Design review of the part built by this model. Coordinates are the model's own, in mm. A direction names the side the tool comes from. Round coordinates to 2 decimals unless told otherwise and drop trailing zeros. Write each loop counter-clockwise with the first axis right and the second up, starting at its lowest first coordinate (ties: lowest second). Pieces come first, ordered by that corner, then holes. Notation, with made-up numbers: (74.25, 4.5) -> (120.25, 4.5) arc R20 ccw to (120.25, 22.5) -> close; hole circle Ø1 at (-18, -6.5). An arc over 180 degrees is marked (long way). Write item = value, one per line. Start each with the question number.
Item 1: For pin 1 Ø1 at (x, z) = (2.5, -11.5) entering from +Y; pin 2 Ø3 at (y, z) = (7, 3.5) entering from +X (3 decimals); pin 3 Ø5 at (y, z) = (-9, 4.5) entering from -X; pin 4 Ø4 at (x, z) = (9.5, 15) entering from +Y, all flat-tipped, find the tip position at first contact; note any pin that passes through.
Item 2: Add section D-D, the plane x = -9. State how many separate pieces and enclosed holes the cut face has, then the cut area to 3 significant figures.
Item 3: Mouldability with a two-part tool opening along Y and no side actions: class faces 1 (the flat face through (0, 0, 21)), 2 (the flat face through (1, -8, 0)), 3 (the cylindrical face through (11.923, 3.755, 0.098)) as released by +Y, released by -Y, zero draft, split by the parting line, or undercut.
Item 4: Machinability: for faces 4 (the flat face through (-2, 4, -14.7)), 5 (the flat face through (-8, 1, 0)), 6 (the cylindrical face through (-4.296, 0.189, 17.894)), which of the approach directions +Z, -Z, +X, -X, +Y, -Y give a long, thin tool a straight path to every point of the face, cutting with its end or side? Answer none if there is none.
Item 5: Add section A-A, the plane z = 5. State the section outline as (x, y) points.
Item 6: To check wall thickness, follow L1, parallel to X at y = -4.5, z = 5; L2, parallel to X at y = -7, z = 2; L3, parallel to Y at x = 0.5, z = -3. State the ranges of each line that lie inside material, in increasing order.
Item 7: Add section B-B, the plane x = 0. State the section outline as (y, z) points, then the cut area to 3 significant figures.
from build123d import *

# Parameters (mm, degrees)
F0_R     = 4.3
F0_R_2   = 2.3
F1_DEPTH = 21
F0_R_3   = 12.5
F2_DEPTH = 14.7


with BuildPart() as f1:
    # F0 (on Top) → F1 (new body, symmetric)
    with BuildSketch(Plane.XY):
        Circle(F0_R)
        Circle(F0_R_2, mode=Mode.SUBTRACT)
        Circle(F0_R_2)
    extrude(amount=F1_DEPTH, both=True)

    # F0 (on Top) → F2 (join, symmetric)
    with BuildSketch(Plane.XY):
        Circle(F0_R_3)
        with BuildLine():
            ThreePointArc((1, 10.4522724802), (7.4246212025, 7.4246212025), (10.4522724802, 1))
            ThreePointArc((10.4522724802, 1), (10.4880613328, 0.5005691551), (10.5, 0))
            ThreePointArc((10.5, 0), (10.4880613328, -0.5005691551), (10.4522724802, -1))
            ThreePointArc((10.4522724802, -1), (7.4246212025, -7.4246212025), (1, -10.4522724802))
            ThreePointArc((1, -10.4522724802), (0, -10.5), (-1, -10.4522724802))
            ThreePointArc((-1, -10.4522724802), (-7.4246212025, -7.4246212025), (-10.4522724802, -1))
            ThreePointArc((-10.4522724802, -1), (-10.5, 0), (-10.4522724802, 1))
            ThreePointArc((-10.4522724802, 1), (-7.4246212025, 7.4246212025), (-1, 10.4522724802))
            ThreePointArc((-1, 10.4522724802), (0, 10.5), (1, 10.4522724802))
        make_face(mode=Mode.SUBTRACT)
        with BuildLine():
            ThreePointArc((4.7968739821, -1), (4.8741503112, -0.5026517123), (4.9, 0))
            ThreePointArc((4.9, 0), (4.8741503112, 0.5026517123), (4.7968739821, 1))
            ThreePointArc((4.7968739821, 1), (3.4648232278, 3.4648232278), (1, 4.7968739821))
            ThreePointArc((1, 4.7968739821), (0, 4.9), (-1, 4.7968739821))
            ThreePointArc((-1, 4.7968739821), (-3.4648232278, 3.4648232278), (-4.7968739821, 1))
            ThreePointArc((-4.7968739821, 1), (-4.9, 0), (-4.7968739821, -1))
            ThreePointArc((-4.7968739821, -1), (-3.4648232278, -3.4648232278), (-1, -4.7968739821))
            ThreePointArc((-1, -4.7968739821), (0, -4.9), (1, -4.7968739821))
            ThreePointArc((1, -4.7968739821), (3.4648232278, -3.4648232278), (4.7968739821, -1))
        make_face()
        Circle(F0_R, mode=Mode.SUBTRACT)
        with BuildLine():
            ThreePointArc((-4.7968739821, -1), (-4.9, 0), (-4.7968739821, 1))
            Line((-4.7968739821, 1), (-10.4522724802, 1))
            ThreePointArc((-10.4522724802, 1), (-10.5, 0), (-10.4522724802, -1))
            Line((-10.4522724802, -1), (-4.7968739821, -1))
        make_face()
        with BuildLine():
            Line((1, -10.4522724802), (1, -4.7968739821))
            ThreePointArc((1, -4.7968739821), (0, -4.9), (-1, -4.7968739821))
            Line((-1, -4.7968739821), (-1, -10.4522724802))
            ThreePointArc((-1, -10.4522724802), (0, -10.5), (1, -10.4522724802))
        make_face()
        with BuildLine():
            ThreePointArc((4.7968739821, 1), (4.8741503112, 0.5026517123), (4.9, 0))
            ThreePointArc((4.9, 0), (4.8741503112, -0.5026517123), (4.7968739821, -1))
            Line((4.7968739821, -1), (10.4522724802, -1))
            ThreePointArc((10.4522724802, -1), (10.4880613328, -0.5005691551), (10.5, 0))
            ThreePointArc((10.5, 0), (10.4880613328, 0.5005691551), (10.4522724802, 1))
            Line((10.4522724802, 1), (4.7968739821, 1))
        make_face()
        with BuildLine():
            ThreePointArc((-1, 4.7968739821), (0, 4.9), (1, 4.7968739821))
            Line((1, 4.7968739821), (1, 10.4522724802))
            ThreePointArc((1, 10.4522724802), (0, 10.5), (-1, 10.4522724802))
            Line((-1, 10.4522724802), (-1, 4.7968739821))
        make_face()
    extrude(amount=F2_DEPTH, both=True)

    # F3 (on Front) → F4 (revolve, cut)
    with BuildSketch(Plane.XZ):
        Polygon((-13.4317712075, 14.7), (-13.4317712075, 6.0651027746), (-4.7968739821, 14.7), align=None)
        Polygon((-13.4317712075, -14.7), (-4.7968739821, -14.7), (-13.4317712075, -6.0651027746), align=None)
    revolve(axis=Axis((0, 0, -14.7), (0, 0, 1)), mode=Mode.SUBTRACT)


solid = f1.part
Result set:
q1.pin_1 = 4.47
q1.pin_2 = 11.225
q1.pin_3 = -10.68
q1.pin_4 = through
q2.separate_pieces = 3
q2.enclosed_holes = 0
q2.area = 147 mm²
q3.face_1 = zero draft
q3.face_2 = undercut
q3.face_3 = split by the parting line
q4.face_4 = -Z
q4.face_5 = +Z, -Z
q4.face_6 = +Z
q5.outline = circle Ø25 at (0, 0); hole (-10.45, -1) arc R10.5 ccw to (-1, -10.45) -> (-1, -4.8) arc R4.9 cw to (-4.8, -1) -> close; hole (-10.45, 1) -> (-4.8, 1) arc R4.9 cw to (-1, 4.8) -> (-1, 10.45) arc R10.5 ccw to start; hole (1, -10.45) arc R10.5 ccw to (10.45, -1) -> (4.8, -1) arc R4.9 cw to (1, -4.8) -> close; hole (1, 4.8) arc R4.9 cw to (4.8, 1) -> (10.45, 1) arc R10.5 ccw to (1, 10.45) -> close
q6.L1 = -11.66 to -9.49, -1.94 to 1.94, 9.49 to 11.66
q6.L2 = -10.36 to -7.83, -1 to 1, 7.83 to 10.36
q6.L3 = -12.49 to 12.49
q7.outline = (-12.5, -7) -> (-4.8, -14.7) -> (-4.3, -14.7) -> (-4.3, -21) -> (4.3, -21) -> (4.3, -14.7) -> (4.8, -14.7) -> (12.5, -7) -> (12.5, 7) -> (4.8, 14.7) -> (4.3, 14.7) -> (4.3, 21) -> (-4.3, 21) -> (-4.3, 14.7) -> (-4.8, 14.7) -> (-12.5, 7) -> close
q7.area = 725 mm²
